Verification items for the finished model (mm, model axes). A direction names the side the tool comes from. Coordinates: 2 decimals unless noted, no trailing zeros. Order: outer loops, then holes, each group sorted by start corner. A loop starts at its lowest first (then second) coordinate and runs counter-clockwise, first axis right, second up.
Q1. Cross-section at A-A, the plane z = 0. Record the boundary of the cut face in (x, y).
Q2. Cross-section at B-B, the plane y = -1.5. Record the boundary of the cut face in (x, z), and give its area (3 significant figures).
Q3. Cross-section at C-C, the plane x = 2. Record the boundary of the cut face in (y, z), and give its area (3 significant figures).
Q4. Set-up check for faces 1 (the cylindrical face through (-0.54, 14.79, 2.44)), 2 (the flat face through (0, 30, 0)): record each of +Z, -Z, +X, -X, +Y, -Y from which the full face is reachable in a straight line by a thin tool's end or side.
Q5. Thickness scan on line 1 (Y direction, x = -0.25, z = 3.25); line 2 (X direction, y = 11, z = 0.25). Record the ranges inside material, lowest first.
Q6. Cross-section at D-D, the plane y = 14. Record the boundary of the cut face in (x, z), and give its area (3 significant figures).
from build123d import *

# Parameters (mm, degrees)
SKETCH1_R           = 2.5
BOSS_EXTRUDE1_DEPTH = 30
BOSS_EXTRUDE2_DEPTH = 4


with BuildPart() as part:
    # Sketch1 → Boss-Extrude1 (new body)
    with BuildSketch(Plane(origin=(0, 0, 0), x_dir=(1, 0, 0), z_dir=(0, 1, 0))):
        Circle(SKETCH1_R)
    extrude(amount=BOSS_EXTRUDE1_DEPTH)

    # Sketch2 → Boss-Extrude2 (add)
    with BuildSketch(Plane.XZ):
        Polygon((0, 5.773502692), (-5, 2.886751346), (-5, -2.886751346), (0, -5.773502692), (5, -2.886751346), (5, 2.886751346), align=None)
    extrude(amount=BOSS_EXTRUDE2_DEPTH)


solid = part.part
Check values:
1. outline: (-5, -4) - (5, -4) - (5, 0) - (2.5, 0) - (2.5, 30) - (-2.5, 30) - (-2.5, 0) - (-5, 0) - close
2. outline: (-5, -2.89) - (0, -5.77) - (5, -2.89) - (5, 2.89) - (0, 5.77) - (-5, 2.89) - close
2. area: 86.6 mm2
3. outline: (-4, -4.62) - (0, -4.62) - (0, -1.5) - (30, -1.5) - (30, 1.5) - (0, 1.5) - (0, 4.62) - (-4, 4.62) - close
3. area: 127 mm2
4. face 1: +Y
4. face 2: +Z, -Z, +X, -X, +Y
5. line 1: y = -4 to 0
5. line 2: x = -2.49 to 2.49
6. outline: circle Ø5 at (0, 0)
6. area: 19.6 mm2
